Read the model definition and answer for the solid it produces. Units are mm, in the model's axes. A direction names the side the tool comes from. Coordinates: 2 decimals unless noted, no trailing zeros. Order: outer loops, then holes, each group sorted by start corner. A loop starts at its lowest first (then second) coordinate and runs counter-clockwise, first axis right, second up. Notation, with made-up numbers: M 86,-20 L 142,-20 A6 cw 142,-12 Z; hole C 3,-28.75 d7. An arc over 180 degrees is marked long. One line per question, with ' | ' between items. Start each with the question number.
1) Find section D-D, the plane z = 3.25. Write down the section's boundary in (x, y), plus the area to 3 significant figures.
2) Find section A-A, the plane z = 0. Write down the section's boundary in (x, y) (3 decimals).
3) A tool of negligible diameter and unlimited length cuts with its end or side. For faces 1 (the face through (0.74, 1.23, 2.36)), 2 (the face through (3, 0.2, 0)), 3 (the face through (-3, 2.3, 0)), from which of +Z, -Z, +X, -X, +Y, -Y can it reach the whole face along a straight path? Write none if from no direction.
4) Find section B-B, the plane x = 0. Write down the section's boundary in (y, z) (3 decimals), plus the area to 4 significant figures.
5) Find section C-C, the plane y = 0.75. Write down the section's boundary in (x, z) (3 decimals).
6) Consider probe 1 along X at (y, z) = (2.45, 0) (3 decimals); probe 2 along X at (y, z) = (0.9, 0) (3 decimals); probe 3 along Z at (x, y) = (1.5, 0.9). Determine where each line is inside the solid, lowest interval first.
7) Given P1, Ø1, axis at y = 1.5, z = -1, coming from the +X side; P2, Ø1.5, axis at x = 1, y = 2, coming from the -Z side; P3, Ø1, axis at y = 1.5, z = -2, coming from the +X side, each flat-ended and moving along its own axis, determine where each tip first touches the part or whether it passes through.
from build123d import *

# Parameters (mm, degrees)
SKETCH_1_R          = 4
SKETCH_1_R_2        = 2.475
EXTRUDE_1_DEPTH     = 2.5
SKETCH_2_R          = 3.5
SKETCH_2_R_2        = 3.2
SKETCH_2_R_3        = 2.725
CUT_EXTRUDE_1_DEPTH = 0.2
CUT_EXTRUDE_START   = -0.2
SKETCH_3_R          = 3.5
SKETCH_3_R_2        = 2.725
CUT_EXTRUDE_2_DEPTH = 0.2


with BuildPart() as part:
    # Эскиз1 → Бобышка-Вытянуть1 (new body)
    with BuildSketch(Plane(origin=(0, 0, 0), x_dir=(1, 0, 0), z_dir=(0, 1, 0))):
        with Locations(Location((0, 0, 0), (0, 0, 270))):
            Circle(SKETCH_1_R)
        with Locations(Location((0, 0, 0), (0, 0, 270))):
            Circle(SKETCH_1_R_2, mode=Mode.SUBTRACT)
    extrude(amount=EXTRUDE_1_DEPTH)

    # Эскиз2 → Вырез-Вытянуть1 (cut)
    # profile 1 of 2: a face of its own
    with BuildSketch(Plane(origin=(0, 2.5, 0), x_dir=(1, 0, 0), z_dir=(0, 1, 0))):
        with Locations(Location((0, 0, 0), (0, 0, 270))):
            Circle(SKETCH_2_R)
        Circle(SKETCH_2_R_2, mode=Mode.SUBTRACT)
    # profile 2 of 2: a face of its own
    with BuildSketch(Plane(origin=(0, 2.5, 0), x_dir=(1, 0, 0), z_dir=(0, 1, 0))):
        Circle(SKETCH_2_R_2)
        with Locations(Location((0, 0, 0), (0, 0, 270))):
            Circle(SKETCH_2_R_3, mode=Mode.SUBTRACT)
    extrude(amount=-CUT_EXTRUDE_1_DEPTH, mode=Mode.SUBTRACT)

    # Эскиз3 → Вырез-Вытянуть2 (cut)
    with BuildSketch(Plane.XZ.offset(CUT_EXTRUDE_START)):
        with Locations(Location((0, 0, 0), (0, 0, 90))):
            Circle(SKETCH_3_R)
        with Locations(Location((0, 0, 0), (0, 0, 90))):
            Circle(SKETCH_3_R_2, mode=Mode.SUBTRACT)
    extrude(amount=CUT_EXTRUDE_2_DEPTH, mode=Mode.SUBTRACT)


solid = part.part
Report:
1) outline: M -2.33,0 L -1.3,0 L -1.3,0.2 L 1.3,0.2 L 1.3,0 L 2.33,0 L 2.33,2.5 L 1.3,2.5 L 1.3,2.3 L -1.3,2.3 L -1.3,2.5 L -2.33,2.5 Z | area: 10.6 mm^2
2) outline: M -4,0 L -3.5,0 L -3.5,0.2 L -2.725,0.2 L -2.725,0 L -2.475,0 L -2.475,2.5 L -2.725,2.5 L -2.725,2.3 L -3.5,2.3 L -3.5,2.5 L -4,2.5 Z; M 2.475,0 L 2.725,0 L 2.725,0.2 L 3.5,0.2 L 3.5,0 L 4,0 L 4,2.5 L 3.5,2.5 L 3.5,2.3 L 2.725,2.3 L 2.725,2.5 L 2.475,2.5 Z
3) face 1: +Y, -Y | face 2: -Y | face 3: +Y
4) outline: M 0,-4 L 2.5,-4 L 2.5,-3.5 L 2.3,-3.5 L 2.3,-2.725 L 2.5,-2.725 L 2.5,-2.475 L 0,-2.475 L 0,-2.725 L 0.2,-2.725 L 0.2,-3.5 L 0,-3.5 Z; M 0,2.475 L 2.5,2.475 L 2.5,2.725 L 2.3,2.725 L 2.3,3.5 L 2.5,3.5 L 2.5,4 L 0,4 L 0,3.5 L 0.2,3.5 L 0.2,2.725 L 0,2.725 Z | area: 7.005 mm^2
5) outline: C 0,0 d8; hole C 0,0 d4.95
6) probe 1: x = -4 to -3.5, -2.725 to -2.475, 2.475 to 2.725, 3.5 to 4 | probe 2: x = -4 to -2.475, 2.475 to 4 | probe 3: z = -3.71 to -1.97, 1.97 to 3.71
7) P1: stops at x = 3.97 | P2: stops at z = -3.99 | P3: stops at x = 3.71
